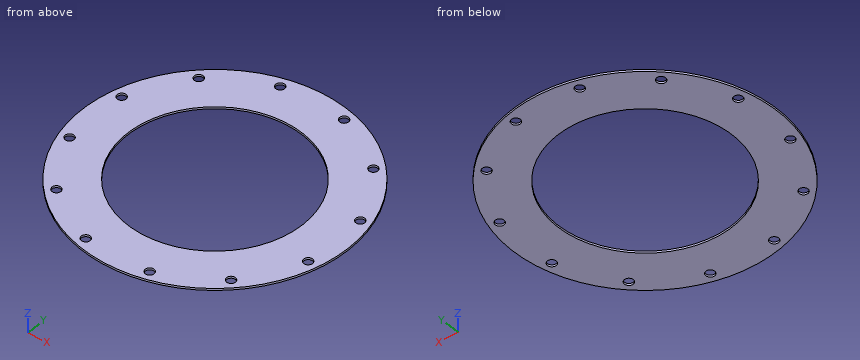
Autodesk Inventor part; units mm, degrees
ref_plane "YZ Plane" through (0, 0, 0) normal (1, 0, 0) x (0, 1, 0)
ref_plane "XZ Plane" through (0, 0, 0) normal (0, 1, 0) x (-1, 0, 0)
ref_plane "XY Plane" through (0, 0, 0) normal (0, 0, 1) x (1, 0, 0)
sketch "スケッチ4" plane through (0, 0, 1) normal (0, 0, 1) x (1, 0, 0)
  circle A0 centre (16.1762, 60.3704) radius 2.25
  circle A1 centre (-16.1762, 60.3704) radius 2.25
  circle A2 centre (0, 0) radius 67.5
  circle A3 centre (-16.1762, 60.3704) radius 5
  circle A4 centre (16.1762, 60.3704) radius 5
  circle A5 centre (0, 0) radius 62.5
  point P0 (-11.2987, 61.4702)
  point P1 (11.2987, 61.4702)
  point P2 (17.4703, 65.2)
  point P3 (-17.4703, 65.2)
sketch "スケッチ1" plane through (0, 0, 0) normal (0, 0, 1) x (1, 0, 0)
  circle A0 centre (0, 0) radius 67.5
  dimension "d0" = 135
extrude "プレート1" add sketch "スケッチ1" along normal blind 1
sketch "スケッチ2" plane through (0, 0, 1) normal (0, 0, 1) x (1, 0, 0)
  circle A0 centre (0, 0) radius 44.5
  dimension "d2" = 89
extrude "押し出し1" cut sketch "スケッチ2" against normal through all
sketch "スケッチ3" plane through (0, 0, 1) normal (0, 0, 1) x (1, 0, 0)
  circle A0 centre (0, 0) radius 62.5
  point P0 (16.1762, 60.3704)
  point P1 (-16.1762, 60.3704)
  point P2 (-44.1942, 44.1942)
  point P3 (-60.3704, 16.1762)
  point P4 (-60.3704, -16.1762)
  point P5 (-44.1942, -44.1942)
  point P6 (-16.1762, -60.3704)
  point P7 (16.1762, -60.3704)
  point P8 (44.1942, -44.1942)
  point P9 (60.3704, -16.1762)
  point P10 (60.3704, 16.1762)
  point P11 (44.1942, 44.1942)
  dimension "d5" = 125
  dimension "d8" = 360
  dimension "d23" = 0
hole "穴1" at (16.1762, 60.3704, 1) at (-16.1762, 60.3704, 1) at (-44.1942, 44.1942, 1) at (-60.3704, 16.1762, 1) at (-60.3704, -16.1762, 1) at (-44.1942, -44.1942, 1) at (-16.1762, -60.3704, 1) at (16.1762, -60.3704, 1) at (44.1942, -44.1942, 1) at (60.3704, -16.1762, 1) at (60.3704, 16.1762, 1) at (44.1942, 44.1942, 1) direction (0, 0, -1) diameter 4.5 end through all
equation "\"d15\" = Thickness"
equation "\"d1\" = Thickness"
equation "\"BendRadius\" = Thickness"
equation "\"BendReliefWidth\" = Thickness"
equation "\"BendReliefDepth\" = 0.5 * Thickness"
equation "\"CornerReliefSize\" = 4 * Thickness"
equation "\"MinimumRemnant\" = 2 * Thickness"
equation "\"TransitionRadius\" = BendRadius"
equation "\"JacobiRadiusSize\" = BendRadius"
equation "\"GapSize\" = Thickness"
properties part number "unit-plate3" material "CFRP"
Here's how the part is built. I have some questions about the finished solid (model axes, mm). Round coordinates to 2 decimals unless told otherwise and drop trailing zeros. Write each loop counter-clockwise with the first axis right and the second up, starting at its lowest first coordinate (ties: lowest second). Pieces come first, ordered by that corner, then holes.
Q1. If we section it at C-C on z = 0.4: Give the number of separate pieces and of enclosed holes in the cut face, plus the area to 3 significant figures.
Q2. If we section it at D-D on x = -49: Write out the boundary of the cut face in (y, z).
Q3. If we section it at A-A on y = 0: Write out the boundary of the cut face in (x, z), plus the area to 3 significant figures.
Q4. Please list where these lines run through material, in increasing order: probe 1 along Y at (x, z) = (60, 0.1); probe 2 along X at (y, z) = (-62, 0.8).
Answer below:
1. separate pieces: 1
1. enclosed holes: 13
1. area: 7,900 mm2
2. outline: (-46.42, 0) - (46.42, 0) - (46.42, 1) - (-46.42, 1) - close
3. outline: (-67.5, 0) - (-44.5, 0) - (-44.5, 1) - (-67.5, 1) - close; (44.5, 0) - (67.5, 0) - (67.5, 1) - (44.5, 1) - close
3. area: 46.0 mm2
4. probe 1: y = -30.92 to -18.4, -13.96 to 13.96, 18.4 to 30.92
4. probe 2: x = -26.69 to -17.73, -14.62 to 14.62, 17.73 to 26.69
